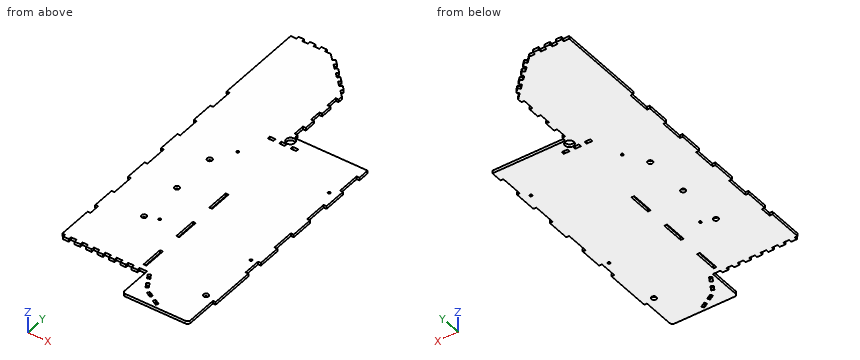
```python
from build123d import *

# Parameters (mm, degrees)
SKETCH1_R           = 4.8895
SKETCH1_R_2         = 1.3335
SKETCH1_R_3         = 2.794
SKETCH1_W           = 3.175
SKETCH1_H           = 25.4
SKETCH1_W_2         = 6.35
SKETCH1_H_2         = 3.175
BOSS_EXTRUDE2_DEPTH = 3.175
FILLET1_R           = 3.175


with BuildPart() as part:
    # Sketch1 → Boss-Extrude2 (new body)
    with BuildSketch(Plane.XY):
        Polygon((0, 3.175), (3.175, 3.175), (3.175, 0), (9.525, 0), (9.525, 3.175), (15.875, 3.175), (15.875, 0), (22.225, 0), (22.225, 3.175), (28.575, 3.175), (28.575, 0), (34.925, 0), (34.925, 3.175), (41.275, 3.175), (41.275, 0), (47.625, 0), (47.625, 3.175), (53.975, 3.175), (53.975, 0), (60.325, 0), (60.325, 3.175), (66.675, 3.175), (66.675, 0), (73.025, 0), (73.025, 3.175), (79.375, 3.175), (79.375, 0), (85.725, 0), (85.725, 3.175), (88.9, 3.175), (94.2848, 3.175), (94.2848, -34.925), (167.535593046, -34.925), (167.535593046, 3.175), (170.4848, 3.175), (170.4848, 53.975), (167.3098, 53.975), (167.3098, 73.025), (170.4848, 73.025), (170.4848, 98.425), (167.3098, 98.425), (167.3098, 123.825), (170.4848, 123.825), (170.4848, 149.225), (167.3098, 149.225), (167.3098, 174.625), (170.4848, 174.625), (170.4848, 200.025), (167.3098, 200.025), (167.3098, 225.425), (170.4848, 225.425), (170.4848, 238.125), (88.9, 238.125), (88.9, 243.205), (85.725, 243.205), (85.725, 255.905), (88.9, 255.905), (88.9, 268.605), (85.725, 268.605), (85.725, 281.305), (88.9, 281.305), (88.9, 294.005), (85.725, 294.005), (85.725, 306.705), (88.9, 306.705), (88.9, 311.785), (82.390448212, 318.294551788), (84.635512242, 320.539615818), (80.145384182, 325.029743879), (77.900320151, 322.784679849), (73.410192091, 327.274807909), (75.655256121, 329.519871939), (71.165128061, 334.01), (68.92006403, 331.76493597), (64.42993597, 336.25506403), (66.675, 338.500128061), (62.184871939, 342.990256121), (59.939807909, 340.745192091), (55.449679849, 345.235320151), (57.694743879, 347.480384182), (53.204615818, 351.970512242), (50.959551788, 349.725448212), (44.45, 356.235), (38.1, 356.235), (38.1, 359.41), (31.75, 359.41), (31.75, 356.235), (25.4, 356.235), (25.4, 359.41), (19.05, 359.41), (19.05, 356.235), (12.7, 356.235), (12.7, 359.41), (6.35, 359.41), (6.35, 356.235), (0, 356.235), (0, 257.175), (3.175, 257.175), (3.175, 231.775), (0, 231.775), (0, 206.375), (3.175, 206.375), (3.175, 180.975), (0, 180.975), (0, 155.575), (3.175, 155.575), (3.175, 130.175), (0, 130.175), (0, 104.775), (3.175, 104.775), (3.175, 79.375), (0, 79.375), (0, 53.975), (3.175, 53.975), (3.175, 42.175), (0, 42.175), (0, 28.575), align=None)
        with Locations((88.9, 232.41)):
            Circle(SKETCH1_R, mode=Mode.SUBTRACT)
        with Locations((59.3598, 191.77)):
            Circle(SKETCH1_R_2, mode=Mode.SUBTRACT)
        with Locations((59.3598, 71.12)):
            Circle(SKETCH1_R_2, mode=Mode.SUBTRACT)
        with Locations((160.9598, 71.12)):
            Circle(SKETCH1_R_2, mode=Mode.SUBTRACT)
        with Locations((160.9598, 191.77)):
            Circle(SKETCH1_R_2, mode=Mode.SUBTRACT)
        with Locations((157.7848, 5.969)):
            Circle(SKETCH1_R_3, mode=Mode.SUBTRACT)
        with Locations((45.225, 66.574999946)):
            Circle(SKETCH1_R_3, mode=Mode.SUBTRACT)
        with Locations((45.225, 117.374999946)):
            Circle(SKETCH1_R_3, mode=Mode.SUBTRACT)
        with Locations((45.225, 168.174999946)):
            Circle(SKETCH1_R_3, mode=Mode.SUBTRACT)
        with Locations((87.3125, 123.825)):
            Rectangle(SKETCH1_W, SKETCH1_H, mode=Mode.SUBTRACT)
        Polygon((99.742302456, 1.4986), (102.917302456, -4.000661314), (100.321651116, -5.499261314), (97.146651116, 0), align=None, mode=Mode.SUBTRACT)
        with Locations((87.3125, 73.025)):
            Rectangle(SKETCH1_W, SKETCH1_H, mode=Mode.SUBTRACT)
        with Locations((87.3125, 22.225)):
            Rectangle(SKETCH1_W, SKETCH1_H, mode=Mode.SUBTRACT)
        with Locations((73.025, 225.0725)):
            Rectangle(SKETCH1_W_2, SKETCH1_H_2, mode=Mode.SUBTRACT)
        with Locations((85.725, 225.0725)):
            Rectangle(SKETCH1_W_2, SKETCH1_H_2, mode=Mode.SUBTRACT)
        with Locations((98.425, 225.0725)):
            Rectangle(SKETCH1_W_2, SKETCH1_H_2, mode=Mode.SUBTRACT)
        Polygon((106.092302456, -9.499922628), (103.496651116, -10.998522628), (106.671651116, -16.497783942), (109.267302456, -14.999183942), align=None, mode=Mode.SUBTRACT)
        Polygon((113.854167186, -19.62934866), (112.355567186, -22.225), (117.8548285, -25.4), (119.3534285, -22.80434866), align=None, mode=Mode.SUBTRACT)
        Polygon((124.852689814, -25.97934866), (123.354089814, -28.575), (128.853351128, -31.75), (130.351951128, -29.15434866), align=None, mode=Mode.SUBTRACT)
    extrude(amount=BOSS_EXTRUDE2_DEPTH)

    # Fillet1
    fillet1_edges = [part.edges().sort_by_distance(p)[0] for p in [
        (88.9, 238.125, 1.5875),
        (167.535593046, -34.925, 1.5875),
        (94.2848, -34.925, 1.5875),
    ]]
    fillet(fillet1_edges, radius=FILLET1_R)


solid = part.part
```
Build history of the part. All positions in model axes, mm. Give positions to 0.01 mm unless a question says otherwise; leave off trailing zeros. Order: outer loops, then holes, each group sorted by start corner. A loop starts at its lowest first (then second) coordinate and runs counter-clockwise, first axis right, second up. Notation, with made-up numbers: M 16.5,12 L 22.5,12 A14 ccw 22.5,36 Z; hole C -11,-12.5 d4. An arc over 180 degrees is marked long. Return JSON: item names as keys, results as strings.
Q1. Band-saw the part on A-A (x = 134). Give the cut face in (y, z) (3 decimals), then the cut area to 3 significant figures.
Answer list:
{"outline": "M -34.925,0 L 238.125,0 L 238.125,3.175 L -34.925,3.175 Z", "area": "867 mm^2"}
Q2. Wall check: probe 1 along X at (y, z) = (71.12, 0.85) (3 decimals); probe 2 along X at (y, z) = (135, 2.55) (3 decimals); probe 3 along X at (y, z) = (25, 2.25) (3 decimals). Give the ranges that are in metal, low to high. Write a range as from..to.
Answer list:
{"probe 1": "x = 0..58.026, 60.693..85.725, 88.9..159.626, 162.293..167.31", "probe 2": "x = 3.175..85.725, 88.9..170.485", "probe 3": "x = 0..85.725, 88.9..170.485"}
Q3. Band-saw the part on B-B (z = 1.7). Count the separate pieces of the cut face and the enclosed holes in it, then the cut area to 3 significant figures.
Answer list:
{"separate pieces": "1", "enclosed holes": "19", "area": "51,300 mm^2"}
Q4. Flat gauge pins, fed straight in: pin 1 (1.6 mm diameter, centred on x = 88, z = 1.5, fed in from +Y) (3 decimals); pin 2 (1.6 mm diameter, centred on x = 99.5, z = 1, fed in from +Y) (3 decimals); pin 3 (1.6 mm diameter, centred on y = 1.5, z = 1, fed in from -X) (3 decimals). Where does each tip first touch, or does it go through?
Answer list:
{"pin 1": "stops at y = 313.485", "pin 2": "stops at y = 238.125", "pin 3": "stops at x = 3.175"}
